Check sheet for the modelled part. Datum: model origin and axes. Units: mm. A direction names the side the tool comes from. Round coordinates to 2 decimals unless told otherwise and drop trailing zeros. Order: outer loops, then holes, each group sorted by start corner. A loop starts at its lowest first (then second) coordinate and runs counter-clockwise, first axis right, second up. Notation, with made-up numbers: (82.5, -29.75) -> (97.5, -29.75) arc R17 ccw to (97.5, -21.75) -> close; hole circle Ø4 at (74.25, 72.25). An arc over 180 degrees is marked (long way). Answer in a Markdown table with one row per item.
```python
from build123d import *

# Parameters (mm, degrees)
SKETCH_1_R      = 1.05
SKETCH_1_R_2    = 1
EXTRUDE_1_DEPTH = 2


with BuildPart() as part:
    # 草图1 → 凸台-拉伸1 (new body)
    with BuildSketch(Plane.XY):
        with BuildLine():
            Line((10, -1.4), (10.5, -1.4))
            ThreePointArc((10.5, -1.4), (10.853553391, -1.253553391), (11, -0.9))
            Line((11, -0.9), (11, 1.1))
            ThreePointArc((11, 1.1), (10.853553391, 1.453553391), (10.5, 1.6))
            Line((10.5, 1.6), (7.5, 1.6))
            ThreePointArc((7.5, 1.6), (7.146446609, 1.746446609), (7, 2.1))
            Line((7, 2.1), (7, 8))
            ThreePointArc((7, 8), (5.602135251, 9.907205584), (3.36256686, 9.148395712))
            Line((3.36256686, 9.148395712), (-2.046791425, 1.435494641))
            ThreePointArc((-2.046791425, 1.435494641), (-2.499635612, -0.042682638), (-1.996588775, -1.504537558))
            Line((-1.996588775, -1.504537558), (2.196410118, -7.068835026))
            ThreePointArc((2.196410118, -7.068835026), (2.931927352, -7.465026056), (3.711498172, -7.164655833))
            Line((3.711498172, -7.164655833), (8.85367593, -1.883782671))
            ThreePointArc((8.85367593, -1.883782671), (9.377885753, -1.525898964), (10, -1.4))
        make_face()
        Circle(SKETCH_1_R, mode=Mode.SUBTRACT)
        with Locations((5, 8)):
            Circle(SKETCH_1_R_2, mode=Mode.SUBTRACT)
    extrude(amount=EXTRUDE_1_DEPTH)


solid = part.part
```
(1) Depth check by flat-ended pin: pin 1 Ø1 at (x, z) = (9, 0.5) entering from +Y; pin 2 Ø1 at (y, z) = (6, 0.5) entering from +X. Enter the tip coordinate at first touch or a pass-through.
Solutions:
| item | result |
|---|---|
| pin 1 | y = 1.6 |
| pin 2 | x = 7 |
(2) Section check D-D on x = 8.5. Record the boundary of the cut face in (y, z).
Solutions:
| item | result |
|---|---|
| outline | (-2.25, 0) -> (1.6, 0) -> (1.6, 2) -> (-2.25, 2) -> close |
(3) Section check A-A on y = 0. Record the boundary of the cut face in (x, z), plus the area to 3 significant figures.
Solutions:
| item | result |
|---|---|
| outline | (-2.5, 0) -> (-1.05, 0) -> (-1.05, 2) -> (-2.5, 2) -> close; (1.05, 0) -> (11, 0) -> (11, 2) -> (1.05, 2) -> close |
| area | 22.8 mm^2 |
(4) Section check B-B on x = 0. Record the boundary of the cut face in (y, z), plus the area to 3 significant figures.
Solutions:
| item | result |
|---|---|
| outline | (-4.15, 0) -> (-1.05, 0) -> (-1.05, 2) -> (-4.15, 2) -> close; (1.05, 0) -> (4.35, 0) -> (4.35, 2) -> (1.05, 2) -> close |
| area | 12.8 mm^2 |
(5) Draft check along X on faces 3 (the cylindrical face through (5, 9, 1)), 4 (the cylindrical face through (2.92, -7.464, 0.986)), 5 (the flat face through (9, 1.6, 1)), 6 (the cylindrical face through (-2.5, 0, 1)). Enter one of: pulls with the +X half, pulls with the -X half, needs draft (parallel to the pull), parting line crosses it, or undercut.
Solutions:
| item | result |
|---|---|
| face 3 | undercut |
| face 4 | parting line crosses it |
| face 5 | needs draft |
| face 6 | pulls with the -X half |
(6) Section check C-C on z = 1.1. Record the boundary of the cut face in (x, y).
Solutions:
| item | result |
|---|---|
| outline | (-2.05, 1.44) arc R2.5 ccw to (-2, -1.5) -> (2.2, -7.07) arc R1 ccw to (3.71, -7.16) -> (8.85, -1.88) arc R1.6 cw to (10, -1.4) -> (10.5, -1.4) arc R0.5 ccw to (11, -0.9) -> (11, 1.1) arc R0.5 ccw to (10.5, 1.6) -> (7.5, 1.6) arc R0.5 cw to (7, 2.1) -> (7, 8) arc R2 ccw to (3.36, 9.15) -> close; hole circle Ø2.1 at (0, 0); hole circle Ø2 at (5, 8) |
(7) Scan lines: probe 1 along Y at (x, z) = (5, 1.55); probe 2 along Y at (x, z) = (0.5, 0.9); probe 3 along X at (y, z) = (-0.75, 0.8). Record each from-to range of solid material in increasing order. Write a range as from..to.
Solutions:
| item | result |
|---|---|
| probe 1 | -5.84..7, 9..10 |
| probe 2 | -4.82..-0.92, 0.92..5.07 |
| probe 3 | -2.38..-0.73, 0.73..11 |
(8) Tool access check on faces 1 (the flat face through (0.07, -4.25, 0.99)), 2 (the flat face through (7, 5, 1)). Record the directions out of +Z, -Z, +X, -X, +Y, -Y that give a thin tool (end or side, any length) a straight path to the whole face; none if there is none.
Solutions:
| item | result |
|---|---|
| face 1 | +Z, -Z, -X, -Y |
| face 2 | +Z, -Z, +X, +Y |
